Part model, mm, in its own coordinate system. A direction names the side the tool comes from. Give positions to 0.01 mm unless a question says otherwise; leave off trailing zeros. Write each loop counter-clockwise with the first axis right and the second up, starting at its lowest first coordinate (ties: lowest second). Pieces come first, ordered by that corner, then holes.
```python
from build123d import *

# Parameters (mm, degrees)
CUT_EXTRUDE_1_DEPTH      = 10.5
CUT_EXTRUDE_2_DEPTH      = 52.961524227
CUT_EXTRUDE_2_DEPTH_BACK = 52.961524227
EXTRUDE_1_REACH          = 40.678
SKETCH_4_R               = 5.75
SKETCH_5_R               = 3.25
CUT_EXTRUDE_3_DEPTH      = 52.961524227
SKETCH_6_W               = 0.8
SKETCH_6_H               = 6
EXTRUDE_2_DEPTH          = 0.3
PATTERN_CIRCULAR_1_COUNT = 13


with BuildPart() as part:
    # Sketch 1 → Revolve 1 (revolve)
    with BuildSketch(Plane.XY, mode=Mode.PRIVATE) as revolve_1_sk:
        Polygon((36, 0), (0, 0), (0, -8.25), (6, -8.25), (6, -10), (20, -10), (20, -5.75), (36, -5.75), align=None)
    revolve(revolve_1_sk.sketch.rotate(Axis((50, 0, 0), (-1, 0, 0)), 270), axis=Axis((50, 0, 0), (-1, 0, 0)))

    # Sketch 2 → Cut-Extrude 1 (cut)
    with BuildSketch(Plane(origin=(20, 0, 0), x_dir=(0, 0, -1), z_dir=(1, 0, 0))):
        with BuildLine():
            ThreePointArc((-4.979646072, 2.875), (-2.875, 4.979646072), (0, 5.75))
            Line((0, 5.75), (-2.299080153, 9.732123635))
            ThreePointArc((-2.299080153, 9.732123635), (-5, 8.660254038), (-7.278726225, 6.857123635))
            Line((-7.278726225, 6.857123635), (-4.979646072, 2.875))
        make_face()
        with BuildLine():
            Line((-2.299080153, -9.732123635), (0, -5.75))
            ThreePointArc((0, -5.75), (-2.875, -4.979646072), (-4.979646072, -2.875))
            Line((-4.979646072, -2.875), (-7.278726225, -6.857123635))
            ThreePointArc((-7.278726225, -6.857123635), (-5, -8.660254038), (-2.299080153, -9.732123635))
        make_face()
        with BuildLine():
            Line((10, 0), (5.75, 0))
            ThreePointArc((5.75, 0), (5.554073501, -1.488209509), (4.979646072, -2.875))
            Line((4.979646072, -2.875), (9.577806377, -2.875))
            ThreePointArc((9.577806377, -2.875), (9.893888613, -1.452917105), (10, 0))
        make_face()
        with BuildLine():
            ThreePointArc((4.979646072, 2.875), (5.554073501, 1.488209509), (5.75, 0))
            Line((5.75, 0), (10, 0))
            ThreePointArc((10, 0), (9.893888613, 1.452917105), (9.577806377, 2.875))
            Line((9.577806377, 2.875), (4.979646072, 2.875))
        make_face()
    extrude(amount=-CUT_EXTRUDE_1_DEPTH, mode=Mode.SUBTRACT)


with BuildPart() as body_2:
    # Sketch 1_3 → Revolve 2 (revolve)
    with BuildSketch(Plane.XY, mode=Mode.PRIVATE) as revolve_2_sk:
        Polygon((50, 0), (36, 0), (36, -5.75), (36, -10), (50, -10), align=None)
    revolve(revolve_2_sk.sketch.rotate(Axis((50, 0, 0), (-1, 0, 0)), 270), axis=Axis((50, 0, 0), (-1, 0, 0)))

    # Sketch 3 → Cut-Extrude 2 (cut, two sides: drawn at the far end of the back side and taken through both)
    with BuildSketch(Plane.XY.offset(-CUT_EXTRUDE_2_DEPTH_BACK)):
        Polygon((36, -10), (36, 10), (46.25, 10), align=None)
    extrude(amount=CUT_EXTRUDE_2_DEPTH + CUT_EXTRUDE_2_DEPTH_BACK, mode=Mode.SUBTRACT)

    # Sketch 4 → Extrude 1 (add, up to next)
    with BuildSketch(Plane(origin=(36, 0, 0), x_dir=(0, 0, -1), z_dir=(1, 0, 0)), mode=Mode.PRIVATE) as extrude_1_sk1:
        with Locations(Location((0, 0, 0), (0, 0, 270))):
            Circle(SKETCH_4_R)
    extrude_1_tool1 = extrude(extrude_1_sk1.sketch, amount=EXTRUDE_1_REACH, mode=Mode.PRIVATE) - body_2.part

    add(part.part)  # Extrude 1 merges part
    add(extrude_1_tool1.solids().sort_by_distance((36, 0, 0))[0])

    # Sketch 5 → Cut-Extrude 3 (cut, through all)
    with BuildSketch(Plane(origin=(50, 0, 0), x_dir=(0, 0, -1), z_dir=(1, 0, 0))):
        Circle(SKETCH_5_R)
    extrude(amount=-CUT_EXTRUDE_3_DEPTH, mode=Mode.SUBTRACT)

    # Sketch 6 → Extrude 2 (add)
    with BuildSketch(Plane(origin=(50, 0, 0), x_dir=(0, 0, -1), z_dir=(1, 0, 0))):
        with Locations((0, 6.5)):
            Rectangle(SKETCH_6_W, SKETCH_6_H)
    extrude_2 = extrude(amount=EXTRUDE_2_DEPTH)

    # Pattern Circular 1: Extrude 2 ×13 about axis
    pattern_circular_1_axis = Axis((0, 0, 0), (1, 0, 0))
    for i in range(1, PATTERN_CIRCULAR_1_COUNT):
        add(extrude_2.rotate(pattern_circular_1_axis, i * 360 / PATTERN_CIRCULAR_1_COUNT))


solid = body_2.part
```
1) Two-plate mould, pull along Z, no slides. Class faces 1 (the face through (9.5, 6, 4)), 2 (the face through (50.3, -4.9, 4.3)), 3 (the face through (44.654, -9.915, 1.302)): +Z half, -Z half, draft (parallel to the pull), parting line (faces both ways), or undercut.
Answers follow:
face 1: undercut
face 2: draft
face 3: parting line
2) Saw through at B-B, the plane x = 16.5. Write the cut outline in (y, z) (3 decimals).
Answers follow:
outline: (-9.732, 2.299) arc R10 ccw to (-2.875, -9.578) - (-2.875, -4.98) arc R5.75 ccw to (2.875, -4.98) - (2.875, -9.578) arc R10 ccw to (9.732, 2.299) - (5.75, 0) arc R5.75 ccw to (2.875, 4.98) - (6.857, 7.279) arc R10 ccw to (-6.857, 7.279) - (-2.875, 4.98) arc R5.75 ccw to (-5.75, 0) - close; hole circle Ø6.5 at (0, 0)
3) Pin check, flat tips, straight feed: pin 1 Ø4 at (y, z) = (0, 0) entering from -X; pin 2 Ø1 at (x, y) = (14.5, 2) entering from +Z; pin 3 Ø2.5 at (x, z) = (16.5, -7.5) entering from +Y; pin 4 Ø10 at (x, y) = (43.5, 7.5) entering from -Z. Stop position of each tip, or through.
Answers follow:
pin 1: passes through
pin 2: stops at z = 9.89
pin 3: stops at y = 7.81
pin 4: stops at z = -9.68
4) Wall check: L1, parallel to Z at x = 48.5, y = -0.25; L2, parallel to Y at x = 27, z = 0; L3, parallel to Y at x = 38.5, z = 0. Give the ranges that are in metal, low to high.
Answers follow:
L1: z = -10 to -3.24, 3.24 to 10
L2: y = -5.75 to -3.25, 3.25 to 5.75
L3: y = -10 to -3.25, 3.25 to 5.75
5) 3-axis set-ups, long thin cutter, end or side, ignore diameter. For faces 4 (the face through (50.3, 0.8, 6.5)), 5 (the face through (14.824, -4.838, 6.113)), 6 (the face through (20, -6, -4)), 7 (the face through (14.824, -7.769, 1.166)): which of +Z, -Z, +X, -X, +Y, -Y reach the whole face in a straight line?
Answers follow:
face 4: +Z, -Z, +X, +Y, -Y
face 5: -Y
face 6: -Z, -Y
face 7: none
6) Saw through at D-D, the plane x = 45. Write the cut outline in (y, z).
Answers follow:
outline: (7.56, -6.54) - (7.56, 6.54) arc R10 ccw (long way) to start; hole circle Ø6.5 at (0, 0)
7) Saw through at C-C, the plane x = 27. Write the cut outline in (y, z), then the cut area to 3 significant figures.
Answers follow:
outline: circle Ø11.5 at (0, 0); hole circle Ø6.5 at (0, 0)
area: 70.7 mm2
8) Saw through at A-A, the plane y = 6.25. Write the cut outline in (x, z).
Answers follow:
outline: (0, -5.39) - (6, -5.39) - (6, -7.81) - (20, -7.81) - (20, 0.29) - (9.5, 0.29) - (9.5, 6.93) - (20, 6.93) - (20, 7.81) - (6, 7.81) - (6, 5.39) - (0, 5.39) - close; (44.33, -7.81) - (50, -7.81) - (50, -3.73) - (50.3, -3.73) - (50.3, -2.83) - (50, -2.83) - (50, -0.4) - (50.3, -0.4) - (50.3, 0.4) - (50, 0.4) - (50, 2.83) - (50.3, 2.83) - (50.3, 3.73) - (50, 3.73) - (50, 7.81) - (44.33, 7.81) - close
